from build123d import *

# Parameters (mm, degrees)
F0_R     = 1.5
F1_DEPTH = 28
F2_DEPTH = 5
F3_R     = 1.5
F4_DEPTH = 3


with BuildPart() as f1:
    # F0 (on Top) → F1 (new body)
    with BuildSketch(Plane.XY):
        Polygon((-3.232447, -1.675851), (-0.164893, -3.637307), (3.067553, -1.961455), (3.232447, 1.675851), (0.164893, 3.637307), (-3.067553, 1.961455), align=None)
        Circle(F0_R, mode=Mode.SUBTRACT)
        Circle(F0_R)
    extrude(amount=-F1_DEPTH)

    # F0 (on Top) → F2 (join)
    with BuildSketch(Plane.XY):
        Circle(F0_R)
    extrude(amount=F2_DEPTH)

    # F3 (on face) → F4 (join)
    with BuildSketch(Plane(origin=(0, 0, -28), x_dir=(1, 0, 0), z_dir=(0, 0, -1))):
        Circle(F3_R)
    extrude(amount=F4_DEPTH)


solid = f1.part
Read the model definition and answer for the solid it produces. Units are mm, in the model's axes. A direction names the side the tool comes from. Round coordinates to 2 decimals unless told otherwise and drop trailing zeros. Order: outer loops, then holes, each group sorted by start corner. A loop starts at its lowest first (then second) coordinate and runs counter-clockwise, first axis right, second up.
1) For faces 1 (the face through (-1.5, -0.07, -29.48)), 2 (the face through (3.15, -0.17, -13.8)), 3 (the face through (-1.5, 0.07, 2.46)), determine the directions among +Z, -Z, +X, -X, +Y, -Y from which every point of the face is accessible in a straight line to the end or side of a thin tool.
2) Flat-ended cylindrical pins translate along their axes: pin 1 (1.5 mm diameter, centred on x = -2.5, y = 3, fed in from -Z); pin 2 (1 mm diameter, centred on y = -1, z = -14, fed in from -X). Find the tip coordinate at first contact, or state that the pin passes through.
3) The part is cut by section B-B on y = 0. Write down the section's boundary in (x, z), plus the area to 3 significant figures.
4) The part is cut by section C-C on x = 2.75. Write down the section's boundary in (y, z), plus the area to 3 significant figures.
5) Straight lines are drawn through the part: L1, parallel to Z at x = 1, y = 1.25; L2, parallel to Y at x = 1.25, z = -7; L3, parallel to Y at x = 1.5, z = -5. For each, find the intervals that lie inside material, in ascending order.
6) The part is cut by section A-A on z = -12. Write down the section's boundary in (x, y), plus the area to 3 significant figures.
Resolved:
1. face 1: -Z
1. face 2: +Z, -Z, +X, -Y
1. face 3: +Z
2. pin 1: stops at z = -28
2. pin 2: stops at x = -3.22
3. outline: (-3.16, -28) - (-1.5, -28) - (-1.5, -31) - (1.5, -31) - (1.5, -28) - (3.16, -28) - (3.16, 0) - (1.5, 0) - (1.5, 5) - (-1.5, 5) - (-1.5, 0) - (-3.16, 0) - close
3. area: 201 mm2
4. outline: (-2.13, -28) - (1.98, -28) - (1.98, 0) - (-2.13, 0) - close
4. area: 115 mm2
5. L1: z = -28 to 0
5. L2: y = -2.9 to 2.94
5. L3: y = -2.77 to 2.78
6. outline: (-3.23, -1.68) - (-0.16, -3.64) - (3.07, -1.96) - (3.23, 1.68) - (0.16, 3.64) - (-3.07, 1.96) - close
6. area: 34.4 mm2
